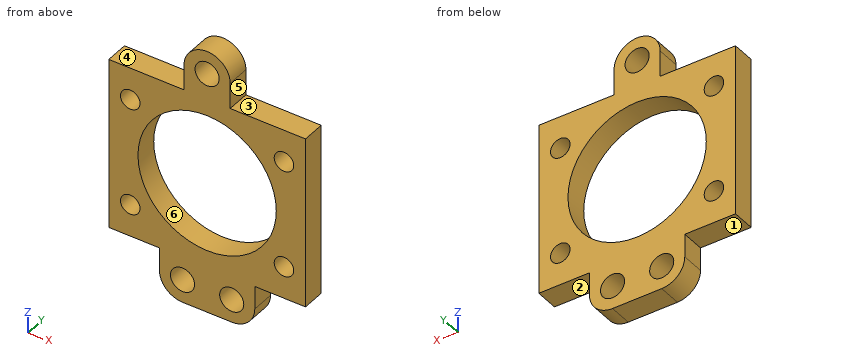
from build123d import *

# Parameters (mm, degrees)
SKETCH1_R              = 44.45
SKETCH1_R_2            = 6.35
BOSS_EXTRUDE1_DEPTH    = 3.175
SKETCH3_R              = 44.45
SKETCH3_R_2            = 27.94
CUT_EXTRUDE2_DEPTH     = 64.181702256
SKETCH7_R              = 2.4892
CUT_EXTRUDE6_DEPTH     = 41.020116192
SKETCH8_R              = 2.0193
CUT_EXTRUDE7_DEPTH     = 41.020116192
CUT_EXTRUDE8_START     = -1.5875
SKETCH9_R              = 27.94
CUT_EXTRUDE8_DEPTH     = 1.5875
CUT_EXTRUDE9_START     = -4.7625
CUT_EXTRUDE9_OUTLINE_R = 27.94
CUT_EXTRUDE9_DEPTH     = 4.7625
SKETCH11_R             = 14.2875
CUT_EXTRUDE10_DEPTH    = 35.823599161


# Read off the part's stored shape, not the designer's step: Cut-Extrude9
with BuildPart() as part:
    # Sketch1 → Boss-Extrude1 (new, symmetric)
    with BuildSketch(Plane(origin=(0, 0, 0), x_dir=(1, 0, 0), z_dir=(0, 1, 0))):
        with Locations(Location((0, 0, 0), (0, 0, 270))):
            Circle(SKETCH1_R)
        with Locations(Location((0, 0, 0), (0, 0, 270))):
            Circle(SKETCH1_R_2, mode=Mode.SUBTRACT)
    extrude(amount=BOSS_EXTRUDE1_DEPTH, both=True)

    # Sketch3 → Cut-Extrude2 (cut, through all)
    with BuildSketch(Plane(origin=(0, 3.175, 0), x_dir=(1, 0, 0), z_dir=(0, 1, 0))):
        Circle(SKETCH3_R)
        with Locations(Location((0, 0, 0), (0, 0, 270))):
            Circle(SKETCH3_R_2, mode=Mode.SUBTRACT)
    extrude(amount=-CUT_EXTRUDE2_DEPTH, mode=Mode.SUBTRACT)

    # Sketch7 → Cut-Extrude6 (cut, through all)
    with BuildSketch(Plane(origin=(0, 3.175, 0), x_dir=(1, 0, 0), z_dir=(0, 1, 0))):
        with Locations(Location((0, -23.114, 0), (0, 0, 270))):
            Circle(SKETCH7_R)
        with Locations(Location((-5.08, 22.548849106, 0), (0, 0, 270))):
            Circle(SKETCH7_R)
        with Locations(Location((5.08, 22.548849106, 0), (0, 0, 270))):
            Circle(SKETCH7_R)
    extrude(amount=-CUT_EXTRUDE6_DEPTH, mode=Mode.SUBTRACT)

    # Sketch8 → Cut-Extrude7 (cut, through all)
    with BuildSketch(Plane.XZ.offset(3.175)):
        with Locations(Location((-15.875, 11.1125, 0), (0, 0, 270))):
            Circle(SKETCH8_R)
        with Locations(Location((15.875, 11.1125, 0), (0, 0, 270))):
            Circle(SKETCH8_R)
        with Locations(Location((15.875, -11.1125, 0), (0, 0, 270))):
            Circle(SKETCH8_R)
        with Locations(Location((-15.875, -11.1125, 0), (0, 0, 270))):
            Circle(SKETCH8_R)
    extrude(amount=-CUT_EXTRUDE7_DEPTH, mode=Mode.SUBTRACT)

    # Sketch9 → Cut-Extrude8 (cut)
    with BuildSketch(Plane.XZ.offset(3.175).offset(CUT_EXTRUDE8_START)):
        with Locations(Location((0, 0, 0), (0, 0, 90))):
            Circle(SKETCH9_R)
    extrude(amount=CUT_EXTRUDE8_DEPTH, mode=Mode.SUBTRACT)

    # Cut-Extrude9 outline → Cut-Extrude9 (cut)
    with BuildSketch(Plane.XZ.offset(1.5875).offset(CUT_EXTRUDE9_START)):
        Circle(CUT_EXTRUDE9_OUTLINE_R)
        with BuildLine():
            Line((-20.32, 17.78), (-4.7625, 17.78))
            Line((-4.7625, 17.78), (-4.7625, 23.114))
            ThreePointArc((-4.7625, 23.114), (0, 27.8765), (4.7625, 23.114))
            Line((4.7625, 23.114), (4.7625, 17.78))
            Line((4.7625, 17.78), (20.32, 17.78))
            Line((20.32, 17.78), (20.32, -17.78))
            Line((20.32, -17.78), (9.8425, -17.78))
            Line((9.8425, -17.78), (9.8425, -22.548849106))
            ThreePointArc((9.8425, -22.548849106), (8.447596045, -25.916445151), (5.08, -27.311349106))
            Line((5.08, -27.311349106), (-5.08, -27.311349106))
            ThreePointArc((-5.08, -27.311349106), (-8.447596045, -25.916445151), (-9.8425, -22.548849106))
            Line((-9.8425, -22.548849106), (-9.8425, -17.78))
            Line((-9.8425, -17.78), (-20.32, -17.78))
            Line((-20.32, -17.78), (-20.32, 17.78))
        make_face(mode=Mode.SUBTRACT)
    extrude(amount=CUT_EXTRUDE9_DEPTH, mode=Mode.SUBTRACT)

    # Sketch11 → Cut-Extrude10 (cut, through all)
    with BuildSketch(Plane.XZ.offset(1.5875)):
        with Locations(Location((0, 0, 0), (0, 0, 270))):
            Circle(SKETCH11_R)
    extrude(amount=-CUT_EXTRUDE10_DEPTH, mode=Mode.SUBTRACT)


solid = part.part
The listing builds one solid part. Answer for the finished solid, in the listing's coordinates (mm). Face numbers are marked on the shaded views. A direction names the side the tool comes from. Coordinates: 2 decimals unless noted, no trailing zeros. Order: outer loops, then holes, each group sorted by start corner. A loop starts at its lowest first (then second) coordinate and runs counter-clockwise, first axis right, second up. Notation, with made-up numbers: (76.25, 14.25) -> (122.25, 14.25) arc R30 ccw to (122.25, 47.25) -> close; hole circle Ø6 at (-23.5, 4.25). An arc over 180 degrees is marked (long way). Answer in a Markdown table with one row per item. Add a question column.
Item 1: Determine the mould class of the marked faces 4, 5 and 6 for opening direction X: +X half, -X half, draft (parallel to the pull), parting line (faces both ways), or undercut.
Item 2: Find section A-A (x = 0). Write down the section's boundary in (y, z) (1 decimal), then the cut area to 3 significant figures.
Item 3: Each of these flat-tipped pins is pushed along its axis until it touches: P1, Ø2.5, axis at x = 15.88, z = -11.11, coming from the +Y side; P2, Ø1.5, axis at x = -11, y = -1, coming from the +Z side; P3, Ø1.4, axis at x = 13, y = 0.5, coming from the -Z side; P4, Ø4.5, axis at x = 15.88, z = 11.11, coming from the +Y side (3 decimals). Where does it stop, or does it pass through?
Item 4: Find section D-D (x = -12). Write down the section's boundary in (y, z) (1 decimal), then the cut area to 3 significant figures.
Item 5: Find section C-C (y = 2.15). State how many separate pieces and enclosed holes the cut face has, then the cut area to 3 significant figures.
Item 6: Which of the six approach directions +Z, -Z, +X, -X, +Y, -Y give full straight-line access (tool end or side, diameter ignored) to the marked faces 1, 2 and 3?
Item 7: Find the intervals of material crossed by L1, parallel to X at y = 0.65, z = 0; L2, parallel to X at y = -1, z = -23; L3, parallel to Z at x = -3, y = 0.85, in increasing order. Write a range as from..to.
Item 8: Find section B-B (z = -6). Write down the section's boundary in (x, y) (1 decimal), then the cut area to 3 significant figures.
Result set:
| question | item | result |
|---|---|---|
| 1 | face 4 | draft |
| 1 | face 5 | +X half |
| 1 | face 6 | undercut |
| 2 | outline | (-1.6, -27.3) -> (3.2, -27.3) -> (3.2, -14.3) -> (-1.6, -14.3) -> close; (-1.6, 14.3) -> (3.2, 14.3) -> (3.2, 20.6) -> (-1.6, 20.6) -> close; (-1.6, 25.6) -> (3.2, 25.6) -> (3.2, 27.9) -> (-1.6, 27.9) -> close |
| 2 | area | 103 mm² |
| 3 | P1 | passes through |
| 3 | P2 | stops at z = 17.78 |
| 3 | P3 | stops at z = -17.78 |
| 3 | P4 | stops at y = 3.175 |
| 4 | outline | (-1.6, -17.8) -> (3.2, -17.8) -> (3.2, -7.8) -> (-1.6, -7.8) -> close; (-1.6, 7.8) -> (3.2, 7.8) -> (3.2, 17.8) -> (-1.6, 17.8) -> close |
| 4 | area | 95.5 mm² |
| 5 | separate pieces | 1 |
| 5 | enclosed holes | 8 |
| 5 | area | 959 mm² |
| 6 | face 1 | -Z, -X, +Y, -Y |
| 6 | face 2 | -Z, +X, +Y, -Y |
| 6 | face 3 | +Z, +X, +Y, -Y |
| 7 | L1 | x = -20.32..-14.29, 14.29..20.32 |
| 7 | L2 | x = -9.82..-7.53, -2.63..2.63, 7.53..9.82 |
| 7 | L3 | z = -27.31..-23.92, -21.18..-13.97, 13.97..26.81 |
| 8 | outline | (-20.3, -1.6) -> (-13, -1.6) -> (-13, 3.2) -> (-20.3, 3.2) -> close; (13, -1.6) -> (20.3, -1.6) -> (20.3, 3.2) -> (13, 3.2) -> close |
| 8 | area | 70.0 mm² |
